Design review of the part built by this model. Coordinates are the model's own, in mm. A direction names the side the tool comes from. Coordinates: 2 decimals unless noted, no trailing zeros. Loops run counter-clockwise (first coordinate to the right, second up) from the corner with the lowest first, then second, coordinate; pieces in that order, holes last. Notation, with made-up numbers: (19, 15) -> (41, 15) arc R30 cw to (41, 38) -> close; hole circle Ø3 at (34.25, 64.5). An arc over 180 degrees is marked (long way). Answer in a Markdown table with one row per item.
Solid Edge part; units mm, degrees
sketch "Sketch1" plane through (0, 0, 0) normal (0, 0, 1) x (1, 0, 0)
  line L0 (-85, -125) -> (85, -125)
  line L1 (85, -125) -> (85, 125)
  line L2 (85, 125) -> (-85, 125)
  line L3 (-85, 125) -> (-85, -125)
  dimension "D1" = 85
  dimension "D2" = 85
extrude "Protrusion1" add sketch "Sketch1" along normal blind 3
sketch "Sketch2" plane through (0, 0, 3) normal (0, 0, 1) x (1, 0, 0)
  circle A0 centre (-58, 90) radius 3
  circle A1 centre (58, 90) radius 3
  circle A2 centre (58, -90) radius 3
  circle A3 centre (-58, -90) radius 3
  dimension "D1" = 58
  dimension "D2" = 58
extrude "Cutout1" cut sketch "Sketch2" against normal through all
sketch "Sketch3" plane through (0, 0, 3) normal (0, 0, 1) x (1, 0, 0)
  line L0 (-85, -65) -> (85, -65)
  line L1 (85, -65) -> (85, 65)
  line L2 (85, 65) -> (-85, 65)
  line L3 (-85, 65) -> (-85, -65)
extrude "Extrusionsausprägung_2" add sketch "Sketch3" along normal blind 3
properties material "Nylon, allgemein"
(1) For pin 1 (0.9 mm diameter, centred on x = 14, z = 5, fed in from -Y); pin 2 (1.5 mm diameter, centred on x = -35, y = -71.5, fed in from +Z); pin 3 (3.5 mm diameter, centred on x = 58, y = 90, fed in from +Z); pin 4 (1 mm diameter, centred on x = 55, z = 4.5, fed in from +Y), all flat-tipped, find the tip position at first contact; note any pin that passes through.
Evaluation:
| item | result |
|---|---|
| pin 1 | stops at y = -65 |
| pin 2 | stops at z = 3 |
| pin 3 | passes through |
| pin 4 | stops at y = 65 |
(2) Take a section at A-A on y = 90. Give the boundary of the cut face in (x, z).
Evaluation:
| item | result |
|---|---|
| outline | (-85, 0) -> (-61, 0) -> (-61, 3) -> (-85, 3) -> close; (-55, 0) -> (55, 0) -> (55, 3) -> (-55, 3) -> close; (61, 0) -> (85, 0) -> (85, 3) -> (61, 3) -> close |
(3) Tool access review of faces 5 (the flat face through (-1, -95, 3)), 6 (the flat face through (-1, 95, 3)), 7 (the cylindrical face through (57.35, 87.07, 1.52)): name each direction out of +Z, -Z, +X, -X, +Y, -Y from which nothing blocks a thin tool from reaching the whole face with its end or side.
Evaluation:
| item | result |
|---|---|
| face 5 | +Z, +X, -X, -Y |
| face 6 | +Z, +X, -X, +Y |
| face 7 | +Z, -Z |
(4) Draft analysis for pull direction X (two halves, no side actions). For faces 1 (the flat face through (-85, 2, 2)), 2 (the flat face through (85, -2, 2)), 3 (the flat face through (-1, 2, 0)), 4 (the cylindrical face through (-58.65, -92.93, 1.52)), state which applies: pulls with the +X half, pulls with the -X half, needs draft (parallel to the pull), parting line crosses it, or undercut.
Evaluation:
| item | result |
|---|---|
| face 1 | pulls with the -X half |
| face 2 | pulls with the +X half |
| face 3 | needs draft |
| face 4 | undercut |
(5) To check wall thickness, follow probe 1 along Y at (x, z) = (-58, 2.35); probe 2 along Y at (x, z) = (-59, 1.6); probe 3 along Z at (x, y) = (55.5, 79). State the ranges of each line that lie inside material, in increasing order.
Evaluation:
| item | result |
|---|---|
| probe 1 | y = -125 to -93, -87 to 87, 93 to 125 |
| probe 2 | y = -125 to -92.83, -87.17 to 87.17, 92.83 to 125 |
| probe 3 | z = 0 to 3 |
(6) Take a section at C-C on x = -48. Give the boundary of the cut face in (y, z), and give its area (3 significant figures).
Evaluation:
| item | result |
|---|---|
| outline | (-125, 0) -> (125, 0) -> (125, 3) -> (65, 3) -> (65, 6) -> (-65, 6) -> (-65, 3) -> (-125, 3) -> close |
| area | 1,140 mm² |
(7) Take a section at D-D on z = 5.05. Give the boundary of the cut face in (x, y), and give its area (3 significant figures).
Evaluation:
| item | result |
|---|---|
| outline | (-85, -65) -> (85, -65) -> (85, 65) -> (-85, 65) -> close |
| area | 22,100 mm² |
(8) Take a section at B-B on x = 58. Give the boundary of the cut face in (y, z), and give its area (3 significant figures).
Evaluation:
| item | result |
|---|---|
| outline | (-125, 0) -> (-93, 0) -> (-93, 3) -> (-125, 3) -> close; (-87, 0) -> (87, 0) -> (87, 3) -> (65, 3) -> (65, 6) -> (-65, 6) -> (-65, 3) -> (-87, 3) -> close; (93, 0) -> (125, 0) -> (125, 3) -> (93, 3) -> close |
| area | 1,100 mm² |
